from build123d import *

# Parameters (mm, degrees)
SKETCH1_W           = 2.1
SKETCH1_H           = 2.1
BOSS_EXTRUDE1_DEPTH = 2
SKETCH4_W           = 2.2
SKETCH4_H           = 2.2
BOSS_EXTRUDE3_DEPTH = 2
SWEEP4_START        = -1.1
SWEEP4_DEPTH        = 2.2
SKETCH8_W           = 2.2
SKETCH8_H           = 2.2
SKETCH8_W_2         = 2
SKETCH8_H_2         = 2
CUT_EXTRUDE2_DEPTH  = 5
SKETCH9_W           = 2
SKETCH9_H           = 2
CUT_EXTRUDE3_DEPTH  = 2


# Read off the part's stored shape, not the designer's step: Sweep4
with BuildPart() as part:
    # Sketch1 → Boss-Extrude1 (new body)
    with BuildSketch(Plane.XY):
        Rectangle(SKETCH1_W, SKETCH1_H)
    extrude(amount=BOSS_EXTRUDE1_DEPTH)

    # Sketch4 → Boss-Extrude3 (add)
    with BuildSketch(Plane.XY):
        Rectangle(SKETCH4_W, SKETCH4_H)
    extrude(amount=-BOSS_EXTRUDE3_DEPTH)

    # Sweep4 outline → Sweep4 (add)
    with BuildSketch(Plane(origin=(0, 0, 0), x_dir=(1, 0, 0), z_dir=(0, 1, 0)).offset(SWEEP4_START)):
        with BuildLine():
            Line((7.09999865, 11.165148445), (7.09999919, 28.5))
            Line((7.09999919, 28.5), (4.89999919, 28.5))
            Line((4.89999919, 28.5), (4.89999865, 11.165148445))
            ThreePointArc((4.89999865, 11.165148445), (4.099633159, 8.481308894), (1.959999989, 6.674225732))
            ThreePointArc((1.959999989, 6.674225732), (-0.2669663, 4.793384792), (-1.1, 2))
            Line((-1.1, 2), (1.1, 2))
            ThreePointArc((1.1, 2), (1.573685829, 3.588395274), (2.839999687, 4.657893766))
            ThreePointArc((2.839999687, 4.657893766), (5.940285288, 7.276319376), (7.09999865, 11.165148445))
        make_face()
    sweep4 = extrude(amount=SWEEP4_DEPTH)

    # Mirror1: Sweep4 across plane
    add(sweep4.mirror(Plane(origin=(0, 0, 0), x_dir=(0, 0, 1), z_dir=(1, 0, 0))))

    # Sketch8 → Cut-Extrude2 (cut)
    with BuildSketch(Plane(origin=(0, 0, -28.5), x_dir=(-1, 0, 0), z_dir=(0, 0, -1))):
        with Locations((-5.99999919, 0)):
            Rectangle(SKETCH8_W, SKETCH8_H)
        with Locations((-5.99999919, 0)):
            Rectangle(SKETCH8_W_2, SKETCH8_H_2, mode=Mode.SUBTRACT)
    cut_extrude2 = extrude(amount=-CUT_EXTRUDE2_DEPTH, mode=Mode.SUBTRACT)

    # Sketch9 → Cut-Extrude3 (cut)
    with BuildSketch(Plane(origin=(0, 0, -28.5), x_dir=(-1, 0, 0), z_dir=(0, 0, -1))):
        with Locations((-5.99999919, 0)):
            Rectangle(SKETCH9_W, SKETCH9_H)
    cut_extrude3 = extrude(amount=-CUT_EXTRUDE3_DEPTH, mode=Mode.SUBTRACT)

    # Mirror2: Cut-Extrude2, Cut-Extrude3 across plane
    add(cut_extrude2.mirror(Plane(origin=(0, 0, 0), x_dir=(0, 0, 1), z_dir=(1, 0, 0))), mode=Mode.SUBTRACT)
    add(cut_extrude3.mirror(Plane(origin=(0, 0, 0), x_dir=(0, 0, 1), z_dir=(1, 0, 0))), mode=Mode.SUBTRACT)


solid = part.part
Read the model definition and answer for the solid it produces. Units are mm, in the model's axes. A direction names the side the tool comes from. Coordinates: 2 decimals unless noted, no trailing zeros. Order: outer loops, then holes, each group sorted by start corner. A loop starts at its lowest first (then second) coordinate and runs counter-clockwise, first axis right, second up. Notation, with made-up numbers: (-38, -35) -> (-18, -35) arc R9 cw to (-18, -23) -> close; hole circle Ø4 at (31, 71.5). An arc over 180 degrees is marked (long way). Answer as a JSON object with one key per item and string values.
1) A tool of negligible diameter and unlimited length cuts with its end or side. For faces 1 (the face through (-1.05, 0, 1)), 2 (the face through (0, 1.05, 1)), 3 (the face through (6, 1, -25)), from which of +Z, -Z, +X, -X, +Y, -Y can it reach the whole face along a straight path? Write none if from no direction.
Model answer:
{"face 1": "+Z, -X, +Y, -Y", "face 2": "+Z, +X, -X, +Y", "face 3": "-Z, +X, -X, +Y"}
2) A cutting plane is placed at A-A, the plane z = -19.25. Determine the outline of the cut face in (x, y), plus the area to 3 significant figures.
Model answer:
{"outline": "(-7.1, -1.1) -> (-4.9, -1.1) -> (-4.9, 1.1) -> (-7.1, 1.1) -> close; (4.9, -1.1) -> (7.1, -1.1) -> (7.1, 1.1) -> (4.9, 1.1) -> close", "area": "9.68 mm²"}
3) A cutting plane is placed at C-C, the plane z = -24.5. Determine the outline of the cut face in (x, y), plus the area to 3 significant figures.
Model answer:
{"outline": "(-7, -1) -> (-5, -1) -> (-5, 1) -> (-7, 1) -> close; (5, -1) -> (7, -1) -> (7, 1) -> (5, 1) -> close", "area": "8.00 mm²"}
4) The mould has two halves that part along X. Classify faces 4 (the face through (-6, 1, -25)), 5 (the face through (-7.1, 0, -17)), 6 (the face through (4.12, -0.02, -8.51)): released by +X, released by -X, zero draft, split by the parting line, or undercut.
Model answer:
{"face 4": "zero draft", "face 5": "released by -X", "face 6": "undercut"}
5) A cutting plane is placed at D-D, the plane x = 2.25. Determine the outline of the cut face in (y, z), plus the area to 3 significant figures.
Model answer:
{"outline": "(-1.1, -6.81) -> (1.1, -6.81) -> (1.1, -4.31) -> (-1.1, -4.31) -> close", "area": "5.50 mm²"}
6) Consider line 1 along X through (y, z) = (0.15, -22.5); line 2 along Z through (x, y) = (5.75, 1.05); line 3 along X through (y, z) = (-0.9, -6.5). Determine where each line is inside the solid, lowest interval first. Write a range as from..to.
Model answer:
{"line 1": "x = -7.1..-4.9, 4.9..7.1", "line 2": "z = -23.5..-7", "line 3": "x = -5.35..-1.6, 1.6..5.35"}
7) Each of these flat-tipped pins is pushed along its axis until it touches: pin 1 (1.6 mm diameter, centred on x = -0.5, z = 1.5, fed in from +Y); pin 2 (2 mm diameter, centred on x = -6, z = -25.5, fed in from +Y); pin 3 (1 mm diameter, centred on y = -0.5, z = -25, fed in from -X); pin 4 (1 mm diameter, centred on x = 3, z = -20.5, fed in from +Y). Where does it stop, or does it pass through?
Model answer:
{"pin 1": "stops at y = 1.05", "pin 2": "stops at y = 1", "pin 3": "stops at x = -7", "pin 4": "passes through"}
